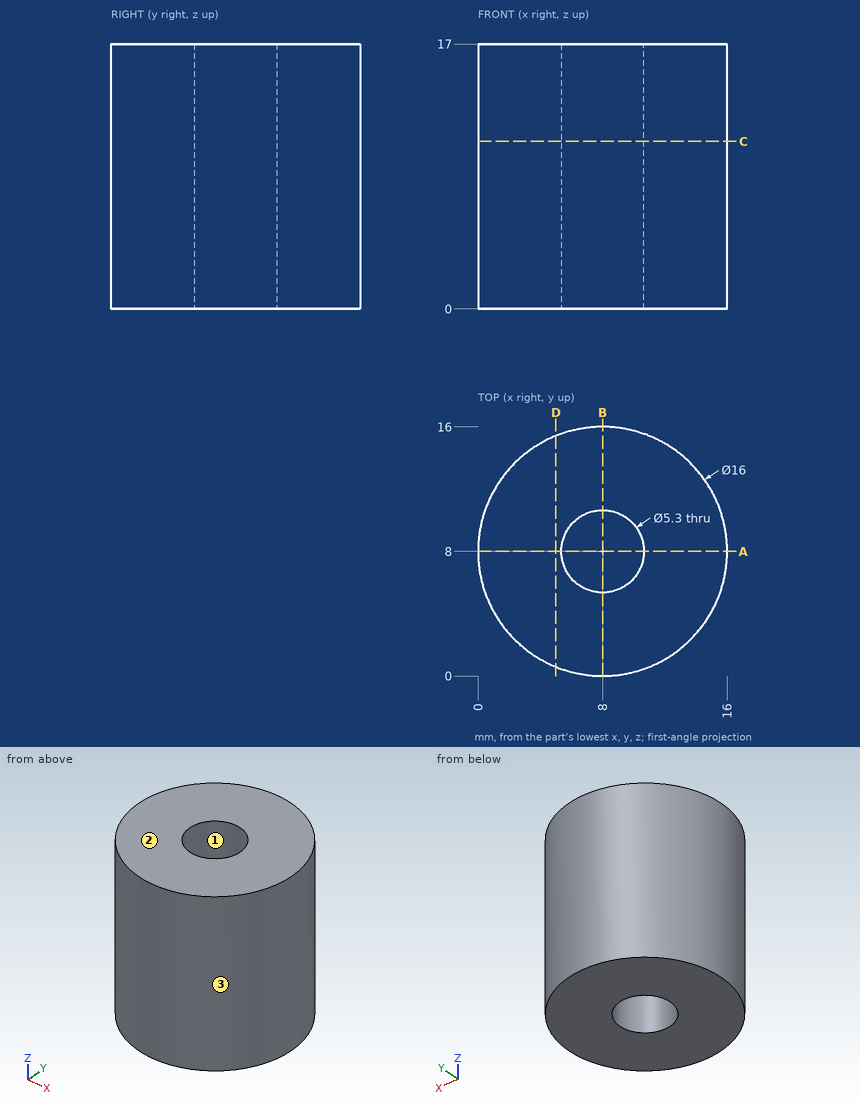
Could you check a few things on this drawing? It's one solid part, dimensions in mm from its lowest x, y, z. Coordinates: 2 decimals unless noted, no trailing zeros. Order: outer loops, then holes, each group sorted by start corner. A loop starts at its lowest first (then second) coordinate and runs counter-clockwise, first axis right, second up.
1. If we section it at A-A (y = 8): Please give me the cut outline in (x, z), then the cut area to 3 significant figures.
2. Thinking about a two-plate mould opening in X: for the marked faces 1, 2 and 3, which applies, +X half, -X half, draft (parallel to the pull), parting line (faces both ways), or undercut?
3. I need wall thicknesses on line 1 (Y direction, x = 8, z = 5); line 2 (X direction, y = 6, z = 3.5); line 3 (X direction, y = 3.5, z = 2). Which ranges of each line are inside material? Lowest first, please.
4. If we section it at D-D (x = 5): Please give me the cut outline in (y, z).
5. If we section it at C-C (z = 10.75): Please give me the cut outline in (x, y).
6. I'm going to push flat-ended pins straight in: pin 1 (1 mm diameter, centred on x = 13, z = 13, fed in from +Y); pin 2 (3 mm diameter, centred on x = 8, y = 8, fed in from +Z); pin 3 (1 mm diameter, centred on y = 13.5, z = 8, fed in from -X) (3 decimals). Where does each tip first touch, or does it pass through?
Entries:
1. outline: (0, 0) - (5.35, 0) - (5.35, 17) - (0, 17) - close; (10.65, 0) - (16, 0) - (16, 17) - (10.65, 17) - close
1. area: 182 mm2
2. face 1: undercut
2. face 2: draft
2. face 3: parting line
3. line 1: y = 0 to 5.35, 10.65 to 16
3. line 2: x = 0.25 to 6.26, 9.74 to 15.75
3. line 3: x = 1.39 to 14.61
4. outline: (0.58, 0) - (15.42, 0) - (15.42, 17) - (0.58, 17) - close
5. outline: circle Ø16 at (8, 8); hole circle Ø5.3 at (8, 8)
6. pin 1: stops at y = 14.61
6. pin 2: passes through
6. pin 3: stops at x = 1.755
